from build123d import *

# Parameters (mm, degrees)
F0_W     = 152.4
F0_H     = 101.6
F1_DEPTH = 50.8
F2_W     = 50.8
F2_H     = 25.4
F3_DEPTH = 50.801
F4_W     = 101.6
F4_H     = 50.8
F4_W_2   = 50.8
F4_H_2   = 25.4
F5_DEPTH = 101.6


with BuildPart() as f1:
    # F0 (on Front) → F1 (new body)
    with BuildSketch(Plane.XZ):
        Rectangle(F0_W, F0_H)
    extrude(amount=F1_DEPTH)

    # F2 (on face) → F3 (cut, through all)
    with BuildSketch(Plane.XZ.offset(50.8)):
        Rectangle(F2_W, F2_H)
    extrude(amount=-F3_DEPTH, mode=Mode.SUBTRACT)

    # F4 (on face) → F5 (join)
    with BuildSketch(Plane.XZ.offset(50.8)):
        Rectangle(F4_W, F4_H)
        Rectangle(F4_W_2, F4_H_2, mode=Mode.SUBTRACT)
    extrude(amount=F5_DEPTH)


solid = f1.part
The listing builds one solid part. Answer for the finished solid, in the listing's coordinates (mm). A direction names the side the tool comes from. Give positions to 0.01 mm unless a question says otherwise; leave off trailing zeros. Loops run counter-clockwise (first coordinate to the right, second up) from the corner with the lowest first, then second, coordinate; pieces in that order, holes last. Notation, with made-up numbers: (40, -15.5) - (64, -15.5) arc R30 ccw to (64, 23.5) - close; hole circle Ø3 at (59.25, 65.5). An arc over 180 degrees is marked (long way). Answer as a JSON object with one key per item and string values.
1. Find the intervals of material crossed by L1, parallel to X at y = -50.5, z = 9; L2, parallel to X at y = -63.5, z = -11.5; L3, parallel to Y at x = 16.5, z = -44, in increasing order. Write a range as [from, to].
Determined:
{"L1": "[-76.2, -25.4], [25.4, 76.2]", "L2": "[-50.8, -25.4], [25.4, 50.8]", "L3": "[-50.8, 0]"}
2. Flat-ended cylindrical pins translate along their axes: pin 1 Ø7.5 at (y, z) = (-90, -4.5) entering from +X; pin 2 Ø12.5 at (y, z) = (-69.5, 5.5) entering from -X; pin 3 Ø15 at (x, y) = (-9, -109.5) entering from -Z. Find the tip coordinate at first contact, or state that the pin passes through.
Determined:
{"pin 1": "x = 50.8", "pin 2": "x = -50.8", "pin 3": "z = -25.4"}
3. For a pull along X with two mould halves and no side action, classify faces 1 (the flat face through (76.2, -25, -1)), 2 (the flat face through (-25.4, -75, 0)), 3 (the flat face through (25.4, -75, 0)), 4 (the flat face through (-1, -50.8, 35)) as pulls with the +X half, pulls with the -X half, needs draft (parallel to the pull), parting line crosses it, or undercut.
Determined:
{"face 1": "pulls with the +X half", "face 2": "undercut", "face 3": "undercut", "face 4": "needs draft"}
4. For faces 5 (the flat face through (0, -75, 12.7)), 6 (the flat face through (-1, -101, -25.4)), 7 (the flat face through (50.8, -101, 0)), 8 (the flat face through (-50.8, -101, 0)), determine the directions among +Z, -Z, +X, -X, +Y, -Y from which every point of the face is accessible in a straight line to the end or side of a thin tool.
Determined:
{"face 5": "+Y, -Y", "face 6": "-Z, +X, -X, -Y", "face 7": "+Z, -Z, +X, -Y", "face 8": "+Z, -Z, -X, -Y"}
5. A cutting plane is placed at D-D (x = -47). Write down the section's boundary in (y, z), then the cut area to 3 significant figures.
Determined:
{"outline": "(-152.4, -25.4) - (-50.8, -25.4) - (-50.8, -50.8) - (0, -50.8) - (0, 50.8) - (-50.8, 50.8) - (-50.8, 25.4) - (-152.4, 25.4) - close", "area": "10,300 mm²"}
6. A cutting plane is placed at B-B (y = -133). Write down the section's boundary in (x, z).
Determined:
{"outline": "(-50.8, -25.4) - (50.8, -25.4) - (50.8, 25.4) - (-50.8, 25.4) - close; hole (-25.4, -12.7) - (25.4, -12.7) - (25.4, 12.7) - (-25.4, 12.7) - close"}
7. A cutting plane is placed at A-A (z = -10). Write down the section's boundary in (x, y), then the cut area to 3 significant figures.
Determined:
{"outline": "(-76.2, -50.8) - (-50.8, -50.8) - (-50.8, -152.4) - (-25.4, -152.4) - (-25.4, 0) - (-76.2, 0) - close; (25.4, -152.4) - (50.8, -152.4) - (50.8, -50.8) - (76.2, -50.8) - (76.2, 0) - (25.4, 0) - close", "area": "10,300 mm²"}
8. A cutting plane is placed at C-C (x = 0). Write down the section's boundary in (y, z), then the cut area to 3 significant figures.
Determined:
{"outline": "(-152.4, -25.4) - (-50.8, -25.4) - (-50.8, -50.8) - (0, -50.8) - (0, -12.7) - (-152.4, -12.7) - close; (-152.4, 12.7) - (0, 12.7) - (0, 50.8) - (-50.8, 50.8) - (-50.8, 25.4) - (-152.4, 25.4) - close", "area": "6,450 mm²"}
